Geometry: see drawing. Coordinates: mm, zero at the bounding-box minimum. A direction names the side the tool comes from. Give positions to 0.01 mm unless a question says otherwise; leave off trailing zeros. Loops run counter-clockwise (first coordinate to the right, second up) from the corner with the lowest first, then second, coordinate; pieces in that order, holes last. Notation, with made-up numbers: M -8.5,-34 L 8.5,-34 A25 ccw 8.5,2 Z; hole C 30.25,-24.5 d3. An arc over 180 degrees is marked long. Answer in a Markdown table with one row per item.
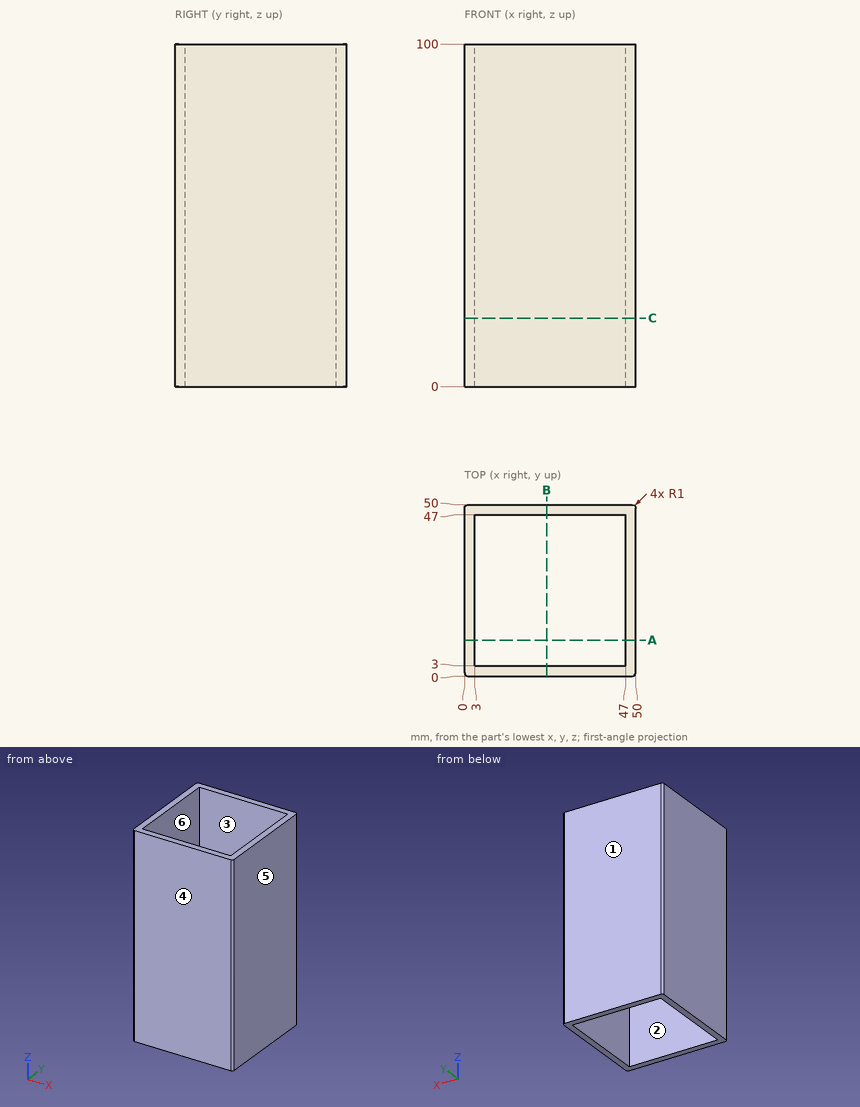
1) Set-up query: the marked faces 5 and 6. Return all of +Z, -Z, +X, -X, +Y, -Y with unobstructed straight access to the full face (end or side cutting, diameter ignored); none if empty.
Reply:
| item | result |
|---|---|
| face 5 | +Z, -Z, +X, +Y, -Y |
| face 6 | +Z, -Z |
2) Pull-direction query (Y, two-part tool) for the marked faces 1, 2, 3 and 4; classes: released by +Y, released by -Y, zero draft, split by the parting line, or undercut.
Reply:
| item | result |
|---|---|
| face 1 | released by +Y |
| face 2 | undercut |
| face 3 | undercut |
| face 4 | released by -Y |
3) Section C-C, the plane z = 20. Return loops of the section in (x, y).
Reply:
| item | result |
|---|---|
| outline | M 0,1 A1 ccw 1,0 L 49,0 A1 ccw 50,1 L 50,49 A1 ccw 49,50 L 1,50 A1 ccw 0,49 Z; hole M 3,3 L 47,3 L 47,47 L 3,47 Z |
4) Section A-A, the plane y = 10.5. Return loops of the section in (x, z), then the cut area to 3 significant figures.
Reply:
| item | result |
|---|---|
| outline | M 0,0 L 3,0 L 3,100 L 0,100 Z; M 47,0 L 50,0 L 50,100 L 47,100 Z |
| area | 600 mm² |
5) Material intervals for L1, parallel to Y at x = 18.5, z = 12, sorted ascending.
Reply:
| item | result |
|---|---|
| L1 | y = 0 to 3, 47 to 50 |
6) Pin query (flat end, axial travel): pin 1 Ø3 at (x, y) = (44, 8) entering from +Z. Return the tip coordinate at first contact, or that it passes through.
Reply:
| item | result |
|---|---|
| pin 1 | passes through |
